CAD build for the part. Positions are in the model's coordinates, mm. Face numbers are marked on the shaded views. A direction names the side the tool comes from. Give positions to 0.01 mm unless a question says otherwise; leave off trailing zeros. Order: outer loops, then holes, each group sorted by start corner. A loop starts at its lowest first (then second) coordinate and runs counter-clockwise, first axis right, second up.
Item 1: Band-saw the part on A-A on y = 27.5. Give the cut face in (x, z), plus the area to 3 significant figures.
Item 2: Band-saw the part on C-C on z = 104. Give the cut face in (x, y).
Item 3: Wall check: L1, parallel to Z at x = -114, y = 23; L2, parallel to X at y = 24, z = 116.5; L3, parallel to Y at x = -170, z = 107.5. Give the ranges that are in metal, low to high.
Item 4: Band-saw the part on B-B on x = -112. Give the cut face in (y, z), plus the area to 3 significant figures.
Item 5: Flat gauge pins, fed straight in: P1, Ø11, axis at x = -167.5, z = 91, coming from the -Y side; P2, Ø3, axis at x = -166, z = 129, coming from the +Y side; P3, Ø16.5, axis at y = 21, z = 92, coming from the -X side. Where does each tip first touch, or does it go through?
Item 6: Which spindle directions (+Z, -Z, +X, -X, +Y, -Y) get a long thin tool onto all of the face, cutting with end or side? Do the marked faces 1, 2 and 3. Say none if no direction does.
```python
from build123d import *

# Parameters (mm, degrees)
SKETCH018_W      = 100
SKETCH018_H      = 20
EXTRUDE018_DEPTH = 150
SKETCH017_W      = 20
SKETCH017_H      = 100
EXTRUDE017_DEPTH = 20
SKETCH019_W      = 10
SKETCH019_H      = 33.333334
EXTRUDE019_DEPTH = 80


with BuildPart() as extrude018:
    # Sketch018 (on Face2 of Extrude017) → Extrude018 (new body)
    with BuildSketch(Plane.YZ.offset(-163.1)):
        with Locations((18.7, 160)):
            Rectangle(SKETCH018_W, SKETCH018_H)
    extrude(amount=EXTRUDE018_DEPTH)


with BuildPart() as extrude017:
    # Sketch017 (on Face4 of Cut015) → Extrude017 (new body)
    with BuildSketch(Plane.XY.offset(150)):
        with Locations((-173.1, 18.7)):
            Rectangle(SKETCH017_W, SKETCH017_H)
    extrude(amount=EXTRUDE017_DEPTH)


with BuildPart() as fusion012:
    # Sketch019 (on Face5 of Extrude017) → Extrude019 (new body)
    with BuildSketch(Plane(origin=(0, 0, 150), x_dir=(1, 0, 0), z_dir=(0, 0, -1))):
        with Locations((-168.1, -18.7)):
            Rectangle(SKETCH019_W, SKETCH019_H)
    extrude(amount=EXTRUDE019_DEPTH)

    # Fusion012: union Extrude018, Extrude017
    add(extrude018.part)
    add(extrude017.part)


solid = fusion012.part
```
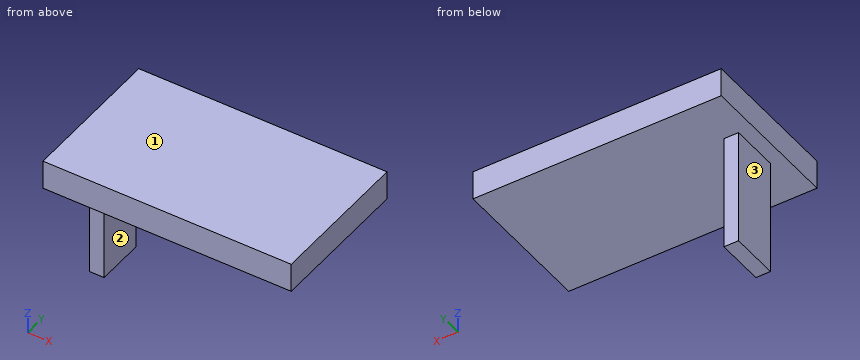
The answers:
1. outline: (-183.1, 150) - (-173.1, 150) - (-173.1, 70) - (-163.1, 70) - (-163.1, 150) - (-13.1, 150) - (-13.1, 170) - (-183.1, 170) - close
1. area: 4,200 mm2
2. outline: (-173.1, 2.03) - (-163.1, 2.03) - (-163.1, 35.37) - (-173.1, 35.37) - close
3. L1: z = 150 to 170
3. L2: x = -173.1 to -163.1
3. L3: y = 2.03 to 35.37
4. outline: (-31.3, 150) - (68.7, 150) - (68.7, 170) - (-31.3, 170) - close
4. area: 2,000 mm2
5. P1: stops at y = 2.03
5. P2: stops at y = 35.37
5. P3: stops at x = -173.1
6. face 1: +Z, +X, -X, +Y, -Y
6. face 2: -Z, +X, +Y, -Y
6. face 3: -Z, -X, +Y, -Y
